```python
from build123d import *

# Parameters (mm, degrees)
SKETCH1_R           = 2
SKETCH1_R_2         = 1.6
BOSS_EXTRUDE1_DEPTH = 7
FILLET1_R           = 10
CUT_EXTRUDE1_DEPTH  = 7


with BuildPart() as part:
    # Sketch1 → Boss-Extrude1 (new body)
    with BuildSketch(Plane(origin=(0, 0, 0), x_dir=(1, 0, 0), z_dir=(0, 1, 0))):
        with BuildLine():
            ThreePointArc((-112, -8), (-55.983036626, -6.600102157), (0, -9))
            ThreePointArc((0, -9), (17.983664082, -7.911906937), (36, -8))
            ThreePointArc((36, -8), (44, 0), (36, 8))
            ThreePointArc((36, 8), (17.983664082, 7.911906937), (0, 9))
            ThreePointArc((0, 9), (-55.983036626, 6.600102157), (-112, 8))
            ThreePointArc((-112, 8), (-120, 0), (-112, -8))
        make_face()
        with Locations(Location((-112, 0, 0), (0, 0, 270))):
            Circle(SKETCH1_R, mode=Mode.SUBTRACT)
        with Locations(Location((0, 0, 0), (0, 0, 270))):
            Circle(SKETCH1_R, mode=Mode.SUBTRACT)
        with Locations(Location((36, 0, 0), (0, 0, 270))):
            Circle(SKETCH1_R_2, mode=Mode.SUBTRACT)
    extrude(amount=BOSS_EXTRUDE1_DEPTH)

    # Fillet1
    fillet1_edges = [part.edges().sort_by_distance(p)[0] for p in [
        (0, 3.5, 9),
        (0, 3.5, -9),
    ]]
    fillet(fillet1_edges, radius=FILLET1_R)

    # Sketch2 → Cut-Extrude1 (cut)
    with BuildSketch(Plane(origin=(0, 7, 0), x_dir=(1, 0, 0), z_dir=(0, 1, 0))):
        with BuildLine():
            Line((-99.309344494, 2.524246591), (-87.854034524, 2.524246591))
            ThreePointArc((-87.854034524, 2.524246591), (-85.329787933, 0), (-87.854034524, -2.524246591))
            Line((-87.854034524, -2.524246591), (-99.309344494, -2.524246591))
            ThreePointArc((-99.309344494, -2.524246591), (-101.833591085, 0), (-99.309344494, 2.524246591))
        make_face()
        with BuildLine():
            Line((-49.629473884, 2.524246591), (-36.48601297, 2.524246591))
            ThreePointArc((-36.48601297, 2.524246591), (-33.96176638, 0), (-36.48601297, -2.524246591))
            Line((-36.48601297, -2.524246591), (-49.629473884, -2.524246591))
            ThreePointArc((-49.629473884, -2.524246591), (-52.153720475, 0), (-49.629473884, 2.524246591))
        make_face()
        with BuildLine():
            Line((16.328995105, 1.800753329), (23.563927718, 1.800753329))
            ThreePointArc((23.563927718, 1.800753329), (25.364681048, 0), (23.563927718, -1.800753329))
            Line((23.563927718, -1.800753329), (16.328995105, -1.800753329))
            ThreePointArc((16.328995105, -1.800753329), (14.528241776, 0), (16.328995105, 1.800753329))
        make_face()
    extrude(amount=-CUT_EXTRUDE1_DEPTH, mode=Mode.SUBTRACT)


solid = part.part
```
Input: part model. Units: mm. Frame: model coordinates. A direction names the side the tool comes from. Coordinates: 2 decimals unless noted, no trailing zeros. Write each loop counter-clockwise with the first axis right and the second up, starting at its lowest first coordinate (ties: lowest second). Pieces come first, ordered by that corner, then holes.
1) Section A-A on z = 0. Output: boundary loops of the cut face in (x, y).
2) Material intervals for line 1 along Z through (x, y) = (-67, 1.75); line 2 along Z through (x, y) = (-15, 5.75); line 3 along Z through (x, y) = (-101, 5), sorted ascending.
3) Pin query (flat end, axial travel): pin 1 Ø3 at (x, z) = (36, 0) entering from -Y; pin 2 Ø2 at (x, y) = (-62, 3.5) entering from +Z; pin 3 Ø3.5 at (x, y) = (-44, 4) entering from -Z; pin 4 Ø2 at (x, y) = (21.5, 2.5) entering from +Z. Return the tip coordinate at first contact, or that it passes through.
4) Section C-C on x = -62. Output: boundary loops of the cut face in (y, z), and give its area (3 significant figures).
5) Set-up query: faces 5 (the cylindrical face through (18.15, 3.451, 7.907)), 6 (the cylindrical face through (18.643, 3.451, -7.894)), 7 (the flat face through (-43, 4, -2.524)). Return all of +Z, -Z, +X, -X, +Y, -Y with unobstructed straight access to the full face (end or side cutting, diameter ignored); none if empty.
6) Section D-D on x = -105. Output: boundary loops of the cut face in (y, z).
7) Mould query, pull axis Z, two halves, no side actions, for faces 1 (the cylindrical face through (-120, 3, 0)), 2 (the cylindrical face through (14.53, 3.55, 0.04)), 3 (the cylindrical face through (-55.622, 3.451, -6.603)), 4 (the flat face through (-43, 4, 2.524)). Classes: pulls with the +Z half, pulls with the -Z half, needs draft (parallel to the pull), parting line crosses it, or undercut.
8) Section B-B on y = 3.75. State how many separate pieces and enclosed holes the cut face has, and give its area (3 significant figures).
Check result:
1. outline: (-120, 0) - (-114, 0) - (-114, 7) - (-120, 7) - close; (-110, 0) - (-101.83, 0) - (-101.83, 7) - (-110, 7) - close; (-85.33, 0) - (-52.15, 0) - (-52.15, 7) - (-85.33, 7) - close; (-33.96, 0) - (-2, 0) - (-2, 7) - (-33.96, 7) - close; (2, 0) - (14.53, 0) - (14.53, 7) - (2, 7) - close; (25.36, 0) - (34.4, 0) - (34.4, 7) - (25.36, 7) - close; (37.6, 0) - (44, 0) - (44, 7) - (37.6, 7) - close
2. line 1: z = -6.58 to 6.58
2. line 2: z = -7.98 to 7.98
2. line 3: z = -7.42 to -1.87, 1.87 to 7.42
3. pin 1: passes through
3. pin 2: stops at z = 6.57
3. pin 3: stops at z = -6.84
3. pin 4: stops at z = 7.85
4. outline: (0, -6.57) - (7, -6.57) - (7, 6.57) - (0, 6.57) - close
4. area: 92.0 mm2
5. face 5: +Z, +Y, -Y
5. face 6: -Z, +Y, -Y
5. face 7: +Y, -Y
6. outline: (0, -7.62) - (7, -7.62) - (7, 7.62) - (0, 7.62) - close
7. face 1: parting line crosses it
7. face 2: undercut
7. face 3: pulls with the -Z half
7. face 4: undercut
8. separate pieces: 1
8. enclosed holes: 6
8. area: 2,170 mm2
